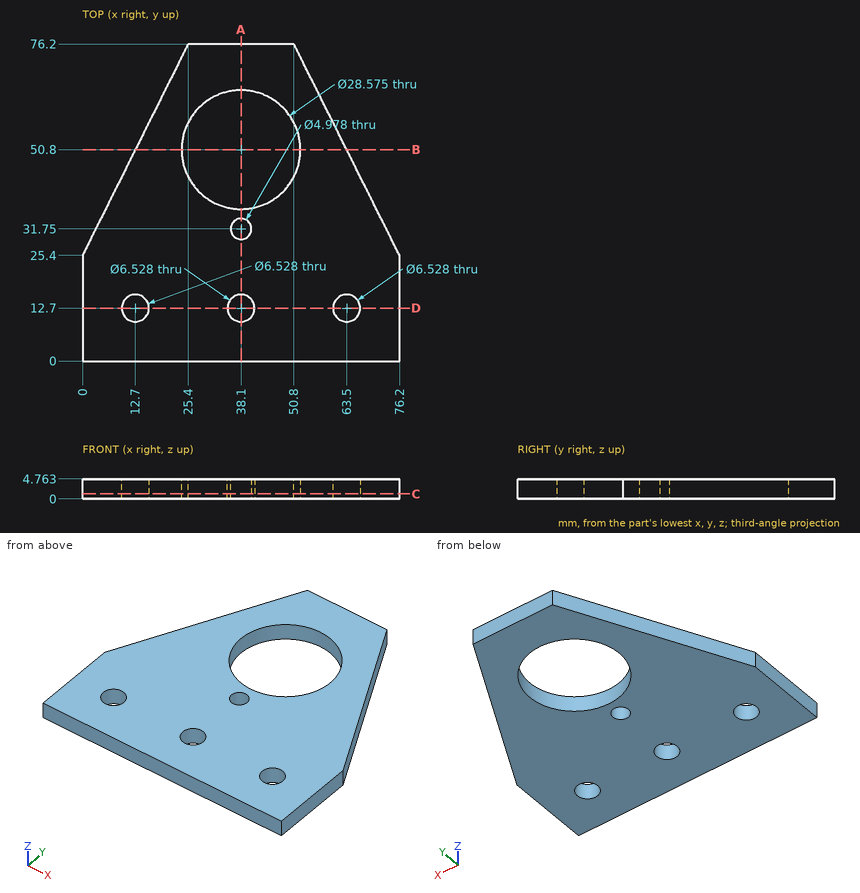
Study the drawing (mm; zero at the part's minimum x, y, z) and answer. Coordinates: 2 decimals unless noted, no trailing zeros. Write each loop counter-clockwise with the first axis right and the second up, starting at its lowest first coordinate (ties: lowest second). Pieces come first, ordered by that corner, then holes. Notation, with made-up numbers: (-17.75, 43.25) - (39.25, 43.25) arc R31 ccw to (39.25, 78.25) - close; hole circle Ø11 at (-29, 27.25). An arc over 180 degrees is marked (long way). Answer as a JSON object with one key per item and string values. Group by question number.
1. A cutting plane is placed at C-C (z = 1.2). Give the number of separate pieces and of enclosed holes in the cut face, plus the area to 4 significant figures.
2. This flat-tipped pin is pushed along its axis until it touches: P1, Ø6, axis at x = 63.5, y = 12.7, coming from the +Z side. Where does it stop, or does it pass through?
3. A cutting plane is placed at B-B (y = 50.8). Determine the outline of the cut face in (x, z), plus the area to 3 significant figures.
4. A cutting plane is placed at D-D (y = 12.7). Determine the outline of the cut face in (x, z).
5. A cutting plane is placed at A-A (x = 38.1). Determine the outline of the cut face in (y, z), plus the area to 3 significant figures.
6. Consider L1, parallel to Y at x = 38.1, z = 2.6; L2, parallel to X at y = 12.7, z = 2.1; L3, parallel to Y at x = 63.5, z = 1.4 (1 decimal). Determine where each line is inside the solid, lowest interval first. Write a range as [from, to].
Worked out:
{
 "1": {"separate pieces": "1", "enclosed holes": "5", "area": "3,755 mm²"},
 "2": {"P1": "passes through"},
 "3": {"outline": "(12.7, 0) - (23.81, 0) - (23.81, 4.76) - (12.7, 4.76) - close; (52.39, 0) - (63.5, 0) - (63.5, 4.76) - (52.39, 4.76) - close", "area": "106 mm²"},
 "4": {"outline": "(0, 0) - (9.44, 0) - (9.44, 4.76) - (0, 4.76) - close; (15.96, 0) - (34.84, 0) - (34.84, 4.76) - (15.96, 4.76) - close; (41.36, 0) - (60.24, 0) - (60.24, 4.76) - (41.36, 4.76) - close; (66.76, 0) - (76.2, 0) - (76.2, 4.76) - (66.76, 4.76) - close"},
 "5": {"outline": "(0, 0) - (9.44, 0) - (9.44, 4.76) - (0, 4.76) - close; (15.96, 0) - (29.26, 0) - (29.26, 4.76) - (15.96, 4.76) - close; (34.24, 0) - (36.51, 0) - (36.51, 4.76) - (34.24, 4.76) - close; (65.09, 0) - (76.2, 0) - (76.2, 4.76) - (65.09, 4.76) - close", "area": "172 mm²"},
 "6": {"L1": "y = [0, 9.44], [15.96, 29.26], [34.24, 36.51], [65.09, 76.2]", "L2": "x = [0, 9.44], [15.96, 34.84], [41.36, 60.24], [66.76, 76.2]", "L3": "y = [0, 9.4], [16, 50.8]"}
}
